from build123d import *

# Parameters (mm, degrees)
SKETCH1_W           = 80
SKETCH1_H           = 90
SKETCH1_R           = 2.1
SKETCH1_W_2         = 19
SKETCH1_H_2         = 53
BOSS_EXTRUDE3_DEPTH = 50
SKETCH5_W           = 70
SKETCH5_H           = 80
CUT_EXTRUDE2_DEPTH  = 45
SKETCH6_R           = 2.5
CUT_EXTRUDE5_DEPTH  = 10.25
CUT_EXTRUDE6_DEPTH  = 10.25
FILLET2_R           = 5
CUT_EXTRUDE9_DEPTH  = 1000


with BuildPart() as part:
    # Sketch1 → Boss-Extrude3 (new body)
    with BuildSketch(Plane(origin=(0, 0, 0), x_dir=(1, 0, 0), z_dir=(0, 1, 0))):
        Rectangle(SKETCH1_W, SKETCH1_H)
        with Locations((29.75, 0)):
            Circle(SKETCH1_R, mode=Mode.SUBTRACT)
        with Locations((-29.75, 0)):
            Circle(SKETCH1_R, mode=Mode.SUBTRACT)
        with Locations((0, -8.5)):
            Rectangle(SKETCH1_W_2, SKETCH1_H_2, mode=Mode.SUBTRACT)
    extrude(amount=BOSS_EXTRUDE3_DEPTH)

    # Sketch5 → Cut-Extrude2 (cut)
    with BuildSketch(Plane(origin=(0, 0, 0), x_dir=(-1, 0, 0), z_dir=(0, -1, 0))):
        Rectangle(SKETCH5_W, SKETCH5_H)
    extrude(amount=-CUT_EXTRUDE2_DEPTH, mode=Mode.SUBTRACT)

    # Sketch6 → Cut-Extrude5 (cut)
    with BuildSketch(Plane(origin=(0, 0, -45), x_dir=(-1, 0, 0), z_dir=(0, 0, -1))):
        with Locations((-5, 40)):
            Circle(SKETCH6_R)
        with Locations((5, 40)):
            Circle(SKETCH6_R)
    extrude(amount=-CUT_EXTRUDE5_DEPTH, mode=Mode.SUBTRACT)

    # Sketch7 → Cut-Extrude6 (cut)
    with BuildSketch(Plane.ZY.offset(40)):
        Polygon((-26.375644347, 31), (-22.334192463, 38), (-26.375644347, 45), (-34.458548116, 45), (-38.5, 38), (-34.458548116, 31), align=None)
        Polygon((34.458548116, 31), (26.375644347, 31), (22.334192463, 38), (26.375644347, 45), (34.458548116, 45), (38.5, 38), align=None)
    extrude(amount=-CUT_EXTRUDE6_DEPTH, mode=Mode.SUBTRACT)

    # Fillet2
    fillet2_edges = [part.edges().sort_by_distance(p)[0] for p in [
        (40, 25, 45),
        (-40, 25, 45),
        (-40, 25, -45),
        (40, 25, -45),
    ]]
    fillet(fillet2_edges, radius=FILLET2_R)

    # Sketch8 → Cut-Extrude9 (cut)
    with BuildSketch(Plane.XY.offset(45)):
        Polygon((-35, 6.24869217), (35, 6.24869217), (35, 4), (30, 4), (30, 0), (-30, 0), (-30, 4), (-35, 4), align=None)
    extrude(amount=-CUT_EXTRUDE9_DEPTH, mode=Mode.SUBTRACT)


solid = part.part
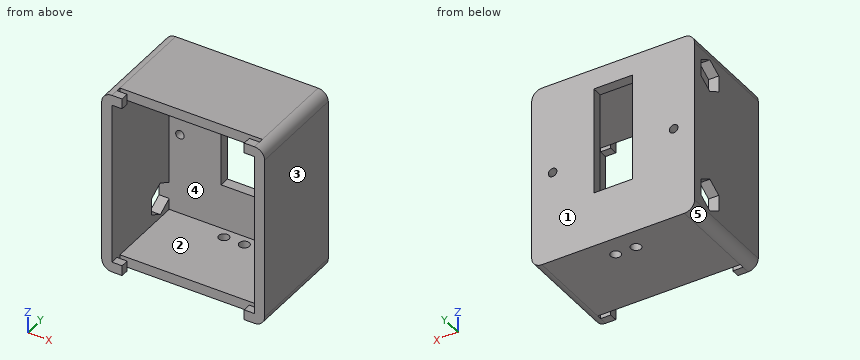
Geometry check sheet. Reference: the model listing, model coordinates, mm. Face numbers are marked on the shaded views. A direction names the side the tool comes from. Give positions to 0.01 mm unless a question says otherwise; leave off trailing zeros. Write each loop counter-clockwise with the first axis right and the second up, starting at its lowest first coordinate (ties: lowest second). Pieces come first, ordered by that corner, then holes. Notation, with made-up numbers: M 13.5,-22.5 L 36.5,-22.5 A24 ccw 36.5,-11.5 Z; hole C 88.5,59 d3. An arc over 180 degrees is marked long. Answer as CSV lines item,"result". Start each with the question number.
Q1. Release check for a two-part mould opening along Z. For the marked faces 3, 4 and 5 record: pulls with the +Z half, pulls with the -Z half, needs draft (parallel to the pull), parting line crosses it, or undercut.
Q2. Section check A-A, the plane x = -5. Record the cut outline in (y, z).
Q3. Section check C-C, the plane y = 16. Record the cut outline in (x, z), then the cut area to 3 significant figures.
Q4. Go/stop test with flat-tipped pins: pin 1 (2.5 mm diameter, centred on x = 29.75, z = 0, fed in from +Y); pin 2 (8 mm diameter, centred on x = -21, z = 28.5, fed in from -Y); pin 3 (5.5 mm diameter, centred on x = 10.5, z = -42, fed in from -Y); pin 4 (1.2 mm diameter, centred on y = 1.5, z = -43.5, fed in from +X). Record where each tip stops, or that it passes through.
Q5. Tool access check on the marked faces 1 and 2. Record the directions out of +Z, -Z, +X, -X, +Y, -Y that give a thin tool (end or side, any length) a straight path to the whole face; none if there is none.
Q6. Material ranges on L1, parallel to X at y = 48.75, z = 0; L2, parallel to Z at x = -2.5, y = 38; L3, parallel to X at y = 38, z = -6.5, recorded low to high.
Q7. Section check B-B, the plane z = 28. Record the cut outline in (x, y), then the cut area to 3 significant figures.
Q8. Section check D-D, the plane z = -31. Record the cut outline in (x, y), then the cut area to 3 significant figures.
Geometry says:
1,face 3,"needs draft"
1,face 4,"undercut"
1,face 5,"pulls with the -Z half"
2,outline,"M 6.25,-45 L 37.5,-45 L 37.5,-40 L 6.25,-40 Z; M 6.25,40 L 45,40 L 45,35 L 50,35 L 50,45 L 6.25,45 Z; M 42.5,-45 L 50,-45 L 50,-18 L 45,-18 L 45,-40 L 42.5,-40 Z"
3,outline,"M -40,-40 A5 ccw -35,-45 L 35,-45 A5 ccw 40,-40 L 40,40 A5 ccw 35,45 L -35,45 A5 ccw -40,40 Z; hole M -35,-40 L 35,-40 L 35,40 L -35,40 Z"
3,area,"1,580 mm^2"
4,pin 1,"through"
4,pin 2,"y = 45"
4,pin 3,"y = 6.25"
4,pin 4,"x = 39.07"
5,face 1,"+Z, -Z, +X, -X, +Y"
5,face 2,"-Y"
6,L1,"-40 to -31.85, -27.65 to -9.5, 9.5 to 27.65, 31.85 to 40"
6,L2,"-45 to -40, 40 to 45"
6,L3,"-40 to -35, 35 to 40"
7,outline,"M -40,0 L -35,0 L -35,31 L -40,31 Z; M -40,45 L -9.5,45 L -9.5,50 L -40,50 Z; M 9.5,45 L 35,45 L 35,0 L 40,0 L 40,50 L 9.5,50 Z"
7,area,"685 mm^2"
8,outline,"M -40,0 L -35,0 L -35,31 L -40,31 Z; M -40,45 L 35,45 L 35,0 L 40,0 L 40,50 L -40,50 Z"
8,area,"780 mm^2"
